For this review, take the finished solid that the model builds, in its own axes (mm). A direction names the side the tool comes from. Round coordinates to 2 decimals unless told otherwise and drop trailing zeros. Order: outer loops, then holes, each group sorted by start corner. A loop starts at its lowest first (then second) coordinate and runs counter-clockwise, first axis right, second up.
```python
from build123d import *

# Parameters (mm, degrees)
F0_R     = 57.15
F0_R_2   = 12.7
F1_DEPTH = 6.35
F2_DEPTH = 285.75
F3_R     = 15.875
F3_R_2   = 12.7
F4_DEPTH = 38.1


with BuildPart() as f1:
    # F0 (on Top) → F1 (new body)
    with BuildSketch(Plane.XY):
        Circle(F0_R)
        Circle(F0_R_2, mode=Mode.SUBTRACT)
        Circle(F0_R_2)
    extrude(amount=F1_DEPTH)

    # F0 (on Top) → F2 (join)
    with BuildSketch(Plane.XY):
        Circle(F0_R)
        Circle(F0_R_2, mode=Mode.SUBTRACT)
    extrude(amount=F2_DEPTH)

    # F3 (on face) → F4 (join)
    with BuildSketch(Plane.XY.offset(285.75)):
        Circle(F3_R)
        Circle(F3_R_2, mode=Mode.SUBTRACT)
    extrude(amount=F4_DEPTH)


solid = f1.part
```
Q1. Wall thickness on line 1 (Y direction, x = 0, z = 186); line 2 (X direction, y = 1, z = 250.5); line 3 (Z direction, x = 45, y = 12): over which ranges is each line inside the solid? List them lowest first.
Q2. Take a section at C-C, the plane z = 23.5. State the section outline as (x, y) points.
Q3. Clearance check with flat-ended pins moving along their axes: pin 1 (10 mm diameter, centred on y = -43.5, z = 87, fed in from -X); pin 2 (4 mm diameter, centred on x = -22.5, z = 156.5, fed in from -Y); pin 3 (6 mm diameter, centred on x = -3.5, z = 69, fed in from -Y). State where each tip first meets the part, or that it passes through.
Q4. Take a section at A-A, the plane y = 0. State the section outline as (x, z) points (3 decimals).
Q5. Tool access review of faces 5 (the face through (-1, 1, 0)), 6 (the face through (12, -12, 285.75)): name each direction out of +Z, -Z, +X, -X, +Y, -Y from which nothing blocks a thin tool from reaching the whole face with its end or side.
Q6. Take a section at D-D, the plane y = -50. State the section outline as (x, z) points, plus the area to 3 significant figures.
Q7. Mouldability with a two-part tool opening along Y and no side actions: class faces 1 (the face through (0, 0, 6.35)), 2 (the face through (-7, 11, 323.85)), 3 (the face through (-3.441, -15.497, 304.533)), 4 (the face through (-2.75, -12.4, 162.88)) as +Y half, -Y half, draft (parallel to the pull), parting line (faces both ways), or undercut.
Working result:
1. line 1: y = -57.15 to -12.7, 12.7 to 57.15
1. line 2: x = -57.14 to -12.66, 12.66 to 57.14
1. line 3: z = 0 to 285.75
2. outline: circle Ø114.3 at (0, 0); hole circle Ø25.4 at (0, 0)
3. pin 1: stops at x = -42.24
3. pin 2: stops at y = -53.35
3. pin 3: stops at y = -57.15
4. outline: (-57.15, 0) - (57.15, 0) - (57.15, 285.75) - (15.875, 285.75) - (15.875, 323.85) - (12.7, 323.85) - (12.7, 6.35) - (-12.7, 6.35) - (-12.7, 323.85) - (-15.875, 323.85) - (-15.875, 285.75) - (-57.15, 285.75) - close
5. face 5: -Z, +X, -X, +Y, -Y
5. face 6: +Z
6. outline: (-27.68, 0) - (27.68, 0) - (27.68, 285.75) - (-27.68, 285.75) - close
6. area: 15,800 mm2
7. face 1: undercut
7. face 2: draft
7. face 3: parting line
7. face 4: undercut
